Can you work these out from the model? Positions are in its coordinate system, mm. A direction names the side the tool comes from. Coordinates: 2 decimals unless noted, no trailing zeros. Write each loop counter-clockwise with the first axis right and the second up, starting at its lowest first coordinate (ties: lowest second). Pieces come first, ordered by that corner, then holes. Notation, with made-up numbers: (-10, 22.5) - (17, 22.5) arc R25 cw to (17, 59.5) - close; hole circle Ø5 at (-4, 70). An arc over 180 degrees is marked (long way). Use one line per item in the form item = value. Start each with the question number.
(1) If I drill on probe 1 along X at (y, z) = (-2.25, -45); probe 2 along Y at (x, z) = (-41, -13); probe 3 along Z at (x, y) = (49.5, -8), over which ranges is the centre line in solid material (lowest first)? Write a range as from..to.
(2) If we section it at C-C on z = 0: Please give me the cut outline in (x, y).
(3) For pin 1 Ø10 at (y, z) = (-21.5, -17) entering from -X; pin 2 Ø8 at (y, z) = (-18, -9) entering from -X; pin 3 Ø1 at (x, z) = (-49.5, -14.5) entering from -Y, each with a flat end and sliding along its axis, tell me the tip position at first contact or that it passes through.
(4) On a 3-axis mill with a long thin cutter (end or side, diameter ignored), from which of +Z, -Z, +X, -X, +Y, -Y can I reach the whole of each face in a straight line? I mean faces 1 (the face through (0, -12, 0)), 2 (the face through (-7, -27, 25)). Say none if no direction works.
(5) Thinking about a two-plate mould opening in Z: for faces 3 (the face through (14, -12, -29)), 4 (the face through (-53.57, -5.92, -41.07)), 5 (the face through (23.846, -19.395, 7.509)), which applies, pulls with the +Z half, pulls with the -Z half, needs draft (parallel to the pull), parting line crosses it, or undercut?
(6) If we section it at A-A on y = -3.5: Please give me the cut outline in (x, z), then the cut area to 3 significant figures.
(7) If we section it at B-B on x = 53: Please give me the cut outline in (y, z).
(8) If we section it at D-D on x = -3: Please give me the cut outline in (y, z).
```python
from build123d import *

# Parameters (mm, degrees)
F0_R     = 67.5
F1_DEPTH = 12
F2_R     = 30
F2_R_2   = 25
F3_DEPTH = 15
F5_DEPTH = 15
F6_COUNT = 5


with BuildPart() as f1:
    # F0 (on Front) → F1 (new body)
    with BuildSketch(Plane.XZ):
        Circle(F0_R)
    extrude(amount=F1_DEPTH)

    # F2 (on face) → F3 (join)
    with BuildSketch(Plane.XZ.offset(12)):
        Circle(F2_R)
        Circle(F2_R_2, mode=Mode.SUBTRACT)
    extrude(amount=F3_DEPTH)

    # F4 (on face) → F5 (cut)
    with BuildSketch(Plane.XZ.offset(12)):
        with BuildLine():
            ThreePointArc((0, 50), (4.9497474683, 52.0502525317), (7, 57))
            ThreePointArc((7, 57), (-4.9497474683, 61.9497474683), (0, 50))
        make_face()
    f5 = extrude(amount=-F5_DEPTH, mode=Mode.SUBTRACT)

    # F6: F5 ×5 about axis
    f6_axis = Axis((0, -12, 0), (0, -1, 0))
    for i in range(1, F6_COUNT):
        add(f5.rotate(f6_axis, i * 360 / F6_COUNT), mode=Mode.SUBTRACT)


solid = f1.part
```
Reported:
q1.probe_1 = -50.31..-40.41, -26.59..26.59, 40.41..50.31
q1.probe_2 = -12..0
q1.probe_3 = -45.89..12.44, 22.79..45.89
q2.outline = (-67.5, -12) - (-30, -12) - (-30, -27) - (-25, -27) - (-25, -12) - (25, -12) - (25, -27) - (30, -27) - (30, -12) - (67.5, -12) - (67.5, 0) - (-67.5, 0) - close
q3.pin_1 = -27.5
q3.pin_2 = -29.58
q3.pin_3 = -12
q4.face_1 = -Y
q4.face_2 = +Z, -Z, +X, -X, -Y
q5.face_3 = needs draft
q5.face_4 = parting line crosses it
q5.face_5 = undercut
q6.outline = circle Ø135 at (0, 0); hole circle Ø14 at (-54.21, 17.61); hole circle Ø14 at (-33.5, -46.11); hole circle Ø14 at (0, 57); hole circle Ø14 at (33.5, -46.11); hole circle Ø14 at (54.21, 17.61)
q6.area = 13,500 mm2
q7.outline = (-12, -41.8) - (0, -41.8) - (0, 10.72) - (-12, 10.72) - close; (-12, 24.51) - (0, 24.51) - (0, 41.8) - (-12, 41.8) - close
q8.outline = (-27, -29.85) - (-12, -29.85) - (-12, -67.43) - (0, -67.43) - (0, 50.68) - (-12, 50.68) - (-12, 29.85) - (-27, 29.85) - (-27, 24.82) - (-12, 24.82) - (-12, -24.82) - (-27, -24.82) - close; (-12, 63.32) - (0, 63.32) - (0, 67.43) - (-12, 67.43) - close
